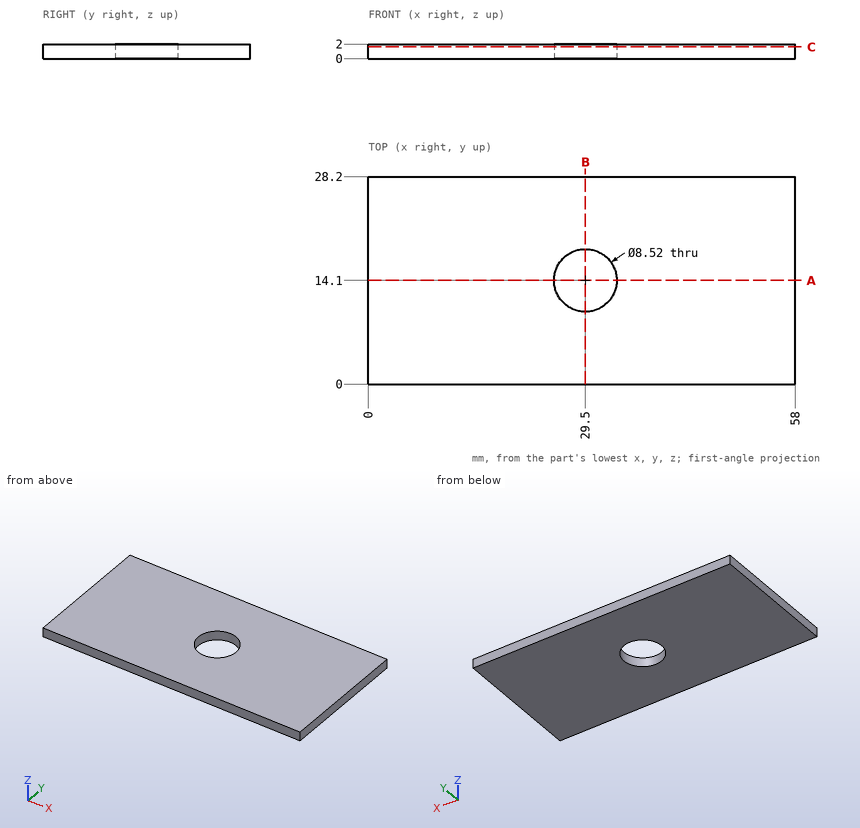
Input: dimensioned drawing with shaded views. Units: mm. Origin: part minimum x, y, z. Give positions to 0.01 mm unless a question says otherwise; leave off trailing zeros. Write each loop counter-clockwise with the first axis right and the second up, starting at its lowest first coordinate (ties: lowest second). Pieces come first, ordered by that corner, then holes. Notation, with made-up numbers: M 37,34 L 94,34 A20 cw 94,73 Z; hole C 50,-7 d5. An arc over 180 degrees is marked long. Return JSON: item names as keys, results as strings. Group by question number.
1) Cut plane A-A, the plane y = 14.1. Output: boundary loops of the cut face in (x, z).
2) Cut plane C-C, the plane z = 1.6. Output: boundary loops of the cut face in (x, y).
3) Material intervals for line 1 along X through (y, z) = (14.1, 0.75); line 2 along Y through (x, z) = (29.5, 0.5); line 3 along Y through (x, z) = (29, 0.55), sorted ascending. Write a range as [from, to].
4) Cut plane B-B, the plane x = 29.5. Output: boundary loops of the cut face in (y, z).
Recorded:
{
 "1": {"outline": "M 0,0 L 25.24,0 L 25.24,2 L 0,2 Z; M 33.76,0 L 58,0 L 58,2 L 33.76,2 Z"},
 "2": {"outline": "M 0,0 L 58,0 L 58,28.2 L 0,28.2 Z; hole C 29.5,14.1 d8.52"},
 "3": {"line 1": "x = [0, 25.24], [33.76, 58]", "line 2": "y = [0, 9.84], [18.36, 28.2]", "line 3": "y = [0, 9.87], [18.33, 28.2]"},
 "4": {"outline": "M 0,0 L 9.84,0 L 9.84,2 L 0,2 Z; M 18.36,0 L 28.2,0 L 28.2,2 L 18.36,2 Z"}
}
